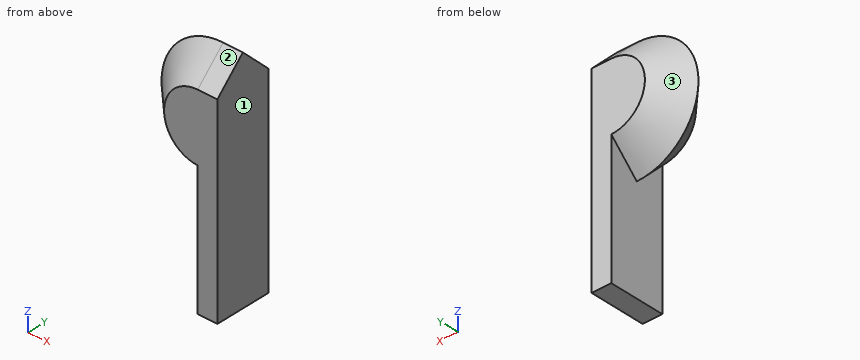
```python
from build123d import *

# Parameters (mm, degrees)
F1_DEPTH = 25.4
F2_SIZE  = 12.69999


# Not quite as in the source:
# - a fillet or chamfer is up to 0.001 mm smaller than in the source, because OpenCascade refuses the exact size


with BuildPart() as f1:
    # F0 (on Front) → F1 (new body)
    with BuildSketch(Plane.XZ):
        with BuildLine():
            Line((8.873289451, 55.7964481413), (0, 55.7964481413))
            ThreePointArc((0, 55.7964481413), (-27.8982240707, 27.8982240707), (0, 0))
            Line((0, 0), (0, -47.0735542476))
            Line((0, -47.0735542476), (8.873289451, -47.0735542476))
            Line((8.873289451, -47.0735542476), (8.873289451, 55.7964481413))
        make_face()
    extrude(amount=F1_DEPTH)

    # F2 (size 12.7 in the source; OpenCascade refuses exactly that, so slightly less here)
    f2_edges = [f1.edges().sort_by_distance(p)[0] for p in [
        (-27.898224, -25.4, 27.898224),
        (-27.898224, 0, 27.898224),
    ]]
    chamfer(f2_edges, length=F2_SIZE)


solid = f1.part
```
Work out the finished part from the listing and answer in its coordinate system (mm). Face numbers are marked on the shaded views. Coordinates: 2 decimals unless noted, no trailing zeros. Loops run counter-clockwise (first coordinate to the right, second up) from the corner with the lowest first, then second, coordinate; pieces in that order, holes last. Notation, with made-up numbers: M 45.5,43 L 96.5,43 A17 ccw 96.5,49 Z; hole C -27,28.5 d10. An arc over 180 degrees is marked long. Use CSV: the item, a comma, the result in double quotes. Start each with the question number.
(1) Consider line 1 (X direction, y = -15.5, z = -20); line 2 (Z direction, x = 6, y = -1.25); line 3 (Z direction, x = 0.5, y = -8.75). Determine where each line is inside the solid, lowest interval first.
(2) Find section D-D, the plane y = -10.25. Give the vertices of the cut face in (x, z).
(3) Given pin 1 Ø5 at (x, y) = (-23, -2.5) entering from -Z; pin 2 Ø3 at (x, z) = (-6.5, 8) entering from -Y, each flat-ended and moving along its own axis, determine where each tip first touches the part or whether it passes through.
(4) Find section B-B, the plane y = -4. Give the vertices of the cut face in (x, z).
(5) For a pull along X with two mould halves and no side action, classify the marked faces 1, 2 and 3 as +X half, -X half, draft (parallel to the pull), parting line (faces both ways), or undercut.
(6) Find section C-C, the plane z = -30.5. Give the vertices of the cut face in (x, y), then the cut area to 3 significant figures.
Recorded:
1,line 1,"x = 0 to 8.87"
1,line 2,"z = -47.07 to 44.35"
1,line 3,"z = -47.07 to 51.85"
2,outline,"M 0,-47.07 L 8.87,-47.07 L 8.87,53.35 L 0,53.35 A25.45 ccw 0,2.45 Z"
3,pin 1,"passes through"
3,pin 2,"stops at y = -21.17"
4,outline,"M 0,-47.07 L 8.87,-47.07 L 8.87,47.1 L 0,47.1 A19.2 ccw 0,8.7 Z"
5,face 1,"+X half"
5,face 2,"draft"
5,face 3,"-X half"
6,outline,"M 0,-25.4 L 8.87,-25.4 L 8.87,0 L 0,0 Z"
6,area,"225 mm^2"
